Geometry check sheet. Reference: the model listing, model coordinates, mm. A direction names the side the tool comes from. Give positions to 0.01 mm unless a question says otherwise; leave off trailing zeros. Loops run counter-clockwise (first coordinate to the right, second up) from the corner with the lowest first, then second, coordinate; pieces in that order, holes last. Notation, with made-up numbers: (67, 13.5) -> (74, 13.5) arc R31 ccw to (74, 44.5) -> close; hole circle Ø2 at (-27, 49). An arc over 180 degrees is marked (long way). One line per item, written item: value. Start each with the question number.
(1) Sectioned sample at D-D, the plane y = 18.5. Record the cut outline in (x, z), then the cut area to 4 significant figures.
(2) Scan lines: line 1 along Y through (x, z) = (0, 17); line 2 along Y through (x, z) = (0, 11); line 3 along Z through (x, y) = (7, 37). Record each from-to range of solid material in increasing order. Write a range as from..to.
(3) Sectioned sample at B-B, the plane y = 39. Record the cut outline in (x, z).
(4) Sectioned sample at A-A, the plane x = 0. Record the cut outline in (y, z), then the cut area to 3 significant figures.
(5) Gauge pin test, flat ends, axial feed: pin 1 Ø16 at (x, z) = (-11.5, 32.5) entering from +Y; pin 2 Ø12 at (x, y) = (0, -21.5) entering from +Z. Record the tip position at first contact, or that the pin passes through.
(6) Tool access check on faces 1 (the face through (0, 46, 6)), 2 (the face through (0, 41, 11.5)). Record the directions out of +Z, -Z, +X, -X, +Y, -Y that give a thin tool (end or side, any length) a straight path to the whole face; none if there is none.
(7) Sectioned sample at C-C, the plane z = 45. Record the cut outline in (x, y), then the cut area to 3 significant figures.
(8) Draft check along Y on faces 3 (the face through (0, 41, 43.5)), 4 (the face through (-1.302, -11.585, 27.115)), 5 (the face through (0, -46, 27)). Enter one of: pulls with the +Y half, pulls with the -Y half, needs draft (parallel to the pull), parting line crosses it, or undercut.
from build123d import *

# Parameters (mm, degrees)
CROQUIS1_W              = 55
CROQUIS1_H              = 92
SALIENTE_EXTRUIR1_DEPTH = 55
CROQUIS2_R              = 10
CORTAR_EXTRUIR1_DEPTH   = 56
CROQUIS3_W              = 32
CROQUIS3_H              = 10.5
CORTAR_EXTRUIR2_DEPTH   = 55


with BuildPart() as part:
    # Croquis1 → Saliente-Extruir1 (new body)
    with BuildSketch(Plane.XY):
        Rectangle(CROQUIS1_W, CROQUIS1_H)
    extrude(amount=SALIENTE_EXTRUIR1_DEPTH)

    # Croquis2 → Cortar-Extruir1 (cut, through all)
    with BuildSketch(Plane.XY):
        with Locations((0, 18.5)):
            Circle(CROQUIS2_R)
        with Locations((0, -21.5)):
            Circle(CROQUIS2_R)
    extrude(amount=CORTAR_EXTRUIR1_DEPTH, mode=Mode.SUBTRACT)

    # Croquis3 → Cortar-Extruir2 (cut)
    with BuildSketch(Plane.ZY.offset(27.5)):
        with Locations((27.5, 40.75)):
            Rectangle(CROQUIS3_W, CROQUIS3_H)
    extrude(amount=-CORTAR_EXTRUIR2_DEPTH, mode=Mode.SUBTRACT)


solid = part.part
Calculated:
1. outline: (-27.5, 0) -> (-10, 0) -> (-10, 55) -> (-27.5, 55) -> close; (10, 0) -> (27.5, 0) -> (27.5, 55) -> (10, 55) -> close
1. area: 1,925 mm2
2. line 1: y = -46..-31.5, -11.5..8.5, 28.5..35.5
2. line 2: y = -46..-31.5, -11.5..8.5, 28.5..46
2. line 3: z = 0..11.5, 43.5..55
3. outline: (-27.5, 0) -> (27.5, 0) -> (27.5, 11.5) -> (-27.5, 11.5) -> close; (-27.5, 43.5) -> (27.5, 43.5) -> (27.5, 55) -> (-27.5, 55) -> close
4. outline: (-46, 0) -> (-31.5, 0) -> (-31.5, 55) -> (-46, 55) -> close; (-11.5, 0) -> (8.5, 0) -> (8.5, 55) -> (-11.5, 55) -> close; (28.5, 0) -> (46, 0) -> (46, 11.5) -> (35.5, 11.5) -> (35.5, 43.5) -> (46, 43.5) -> (46, 55) -> (28.5, 55) -> close
4. area: 2,520 mm2
5. pin 1: stops at y = 35.5
5. pin 2: passes through
6. face 1: +Z, -Z, +X, -X, +Y
6. face 2: +X, -X, +Y
7. outline: (-27.5, -46) -> (27.5, -46) -> (27.5, 46) -> (-27.5, 46) -> close; hole circle Ø20 at (0, -21.5); hole circle Ø20 at (0, 18.5)
7. area: 4,430 mm2
8. face 3: needs draft
8. face 4: undercut
8. face 5: pulls with the -Y half
